Could you check a few things on this model? Use its own coordinates, in mm. A direction names the side the tool comes from. Give positions to 0.01 mm unless a question says otherwise; leave off trailing zeros. Loops run counter-clockwise (first coordinate to the right, second up) from the corner with the lowest first, then second, coordinate; pieces in that order, holes last. Notation, with made-up numbers: (58.5, 55) -> (109.5, 55) arc R30 cw to (109.5, 84) -> close; hole circle Ø7 at (77, 30). An arc over 180 degrees is marked (long way). Write each question's results on one line, items separated by ' | '. Start each with the question number.
Q1. If we section it at C-C, the plane z = 5.75: List the corners of the cut face in (x, y) for me.
Q2. Will these pins go through, and if not, where does the flat tip stop? P1, Ø7, axis at y = -15.5, z = 20.5, coming from the +X side; P2, Ø4, axis at x = -3.5, z = 21.5, coming from the +Y side.
Q3. If I drill on line 1 along X through (y, z) = (-20.9, 10); line 2 along X through (y, z) = (-13, 17.75); line 3 along Y through (x, z) = (-8, 6.25), over which ranges is the centre line in solid material (lowest first)?
Q4. If we section it at B-B, the plane y = -10.59: List the corners of the cut face in (x, z) for me, plus the area to 3 significant figures.
Q5. We'd pull the mould along Z, two halves only. Please class faces 1 (the face through (-0.19, -20.83, 2.75)), 2 (the face through (-6, -21, 0)), 3 (the face through (-9, -14, 30)): released by +Z, released by -Z, zero draft, split by the parting line, or undercut.
Q6. If we section it at A-A, the plane z = 10: List the corners of the cut face in (x, y) for me, plus the area to 4 significant figures.
Q7. If we section it at D-D, the plane x = 1.75: List the corners of the cut face in (y, z) for me.
Q8. Which directions (+Z, -Z, +X, -X, +Y, -Y) give clear straight access to the entire face, cutting with the end or side of a thin tool? Please do faces 4 (the face through (-9.773, -14, 15)), 5 (the face through (-1.6, -20.09, 11.5)).
from build123d import *

# Parameters (mm, degrees)
EXTRUSION1_DEPTH = 30
ESQUISSE3_R      = 1.5
EXTRUSION2_DEPTH = 60
ESQUISSE4_R      = 1.5
EXTRUSION3_DEPTH = 60


with BuildPart() as part:
    # Esquisse1 → Extrusion1 (new body)
    with BuildSketch(Plane.XY):
        Polygon((-9.773002169, -6.59), (-8.273002169, -6.59), (-8.273002169, -20.09), (5.226997831, -20.09), (5.226997831, -21.59), (-9.773002169, -21.59), align=None)
    extrude(amount=EXTRUSION1_DEPTH)

    # Esquisse3 → Extrusion2 (cut)
    with BuildSketch(Plane(origin=(-8.273002169, 0, 0), x_dir=(0, 0, -1), z_dir=(1, 0, 0))):
        with Locations(Location((-24, -10.59, 0), (0, 0, 90))):
            Circle(ESQUISSE3_R)
        with Locations(Location((-24, -17.59, 0), (0, 0, 90))):
            Circle(ESQUISSE3_R)
    extrude(amount=-EXTRUSION2_DEPTH, mode=Mode.SUBTRACT)

    # Esquisse4 → Extrusion3 (cut)
    with BuildSketch(Plane(origin=(0, -20.09, 0), x_dir=(-1, 0, 0), z_dir=(0, 1, 0))):
        with Locations(Location((2.773002169, 10, 0), (0, 0, 90))):
            Circle(ESQUISSE4_R)
        with Locations(Location((-0.726997831, 3.937822174, 0), (0, 0, 90))):
            Circle(ESQUISSE4_R)
        Polygon((-5.226997831, 30), (8.273002169, 30), (-5.226997831, 12), align=None)
    extrude(amount=-EXTRUSION3_DEPTH, mode=Mode.SUBTRACT)


solid = part.part
Final values:
1) outline: (-9.77, -21.59) -> (5.23, -21.59) -> (5.23, -20.09) -> (-8.27, -20.09) -> (-8.27, -6.59) -> (-9.77, -6.59) -> close
2) P1: stops at x = -8.27 | P2: stops at y = -20.09
3) line 1: x = -9.77 to -4.27, -1.27 to 5.23 | line 2: x = -9.77 to -8.27 | line 3: y = -21.59 to -20.09
4) outline: (-9.77, 0) -> (-8.27, 0) -> (-8.27, 22.5) -> (-9.77, 22.5) -> close; (-9.77, 25.5) -> (-8.27, 25.5) -> (-8.27, 30) -> (-9.77, 30) -> close | area: 40.5 mm²
5) face 1: undercut | face 2: released by -Z | face 3: released by +Z
6) outline: (-9.77, -21.59) -> (-4.27, -21.59) -> (-4.27, -20.09) -> (-8.27, -20.09) -> (-8.27, -6.59) -> (-9.77, -6.59) -> close; (-1.27, -21.59) -> (5.23, -21.59) -> (5.23, -20.09) -> (-1.27, -20.09) -> close | area: 38.25 mm²
7) outline: (-21.59, 0) -> (-20.09, 0) -> (-20.09, 2.84) -> (-21.59, 2.84) -> close; (-21.59, 5.03) -> (-20.09, 5.03) -> (-20.09, 16.64) -> (-21.59, 16.64) -> close
8) face 4: +Z, -Z, -X, +Y, -Y | face 5: +Z, -Z, +X, +Y
